```python
from build123d import *

# Parameters (mm, degrees)
SKETCH4_W           = 60
SKETCH4_H           = 40
BOSS_EXTRUDE1_DEPTH = 20
FILLET1_R           = 5
FILLET2_R           = 5
CUT_EXTRUDE1_DEPTH  = 8
CUT_EXTRUDE2_DEPTH  = 8
SKETCH8_R           = 1.5
CUT_EXTRUDE4_DEPTH  = 8
SHELL3_START        = 2
SHELL3_DEPTH        = 18
SKETCH9_W           = 10.049922194
SKETCH9_H           = 4.5
BOSS_EXTRUDE2_DEPTH = 1
SKETCH10_W          = 0.584985694
SKETCH10_H          = 1.811393404
CUT_EXTRUDE5_DEPTH  = 0.1
CUT_EXTRUDE6_DEPTH  = 5.1


# Read off the part's stored shape, not the designer's step: Shell3
with BuildPart() as part:
    # Sketch4 → Boss-Extrude1 (new body)
    with BuildSketch(Plane(origin=(0, 0, 0), x_dir=(1, 0, 0), z_dir=(0, 1, 0))):
        with Locations((-9.826955075, -12.370810554)):
            Rectangle(SKETCH4_W, SKETCH4_H)
    extrude(amount=BOSS_EXTRUDE1_DEPTH)

    # Fillet1
    fillet1_edges = [part.edges().sort_by_distance(p)[0] for p in [
        (20.173044925, 10, 32.370810554),
    ]]
    fillet(fillet1_edges, radius=FILLET1_R)

    # Fillet2
    fillet2_edges = [part.edges().sort_by_distance(p)[0] for p in [
        (20.173044925, 10, -7.629189446),
        (-39.826955075, 10, 32.370810554),
    ]]
    fillet(fillet2_edges, radius=FILLET2_R)

    # Sketch6 → Cut-Extrude1 (cut)
    with BuildSketch(Plane(origin=(0, 20, 0), x_dir=(1, 0, 0), z_dir=(0, 1, 0))):
        Polygon((-32.326955075, 7.629189446), (-39.826955075, 0.129189446), (-39.826955075, 7.629189446), align=None)
    extrude(amount=-CUT_EXTRUDE1_DEPTH, mode=Mode.SUBTRACT)

    # Sketch7 → Cut-Extrude2 (cut)
    with BuildSketch(Plane.XZ):
        Polygon((-32.326955075, -7.629189446), (-39.826955075, -0.129189446), (-39.826955075, -7.629189446), align=None)
    extrude(amount=-CUT_EXTRUDE2_DEPTH, mode=Mode.SUBTRACT)

    # Sketch8 → Cut-Extrude4 (cut)
    with BuildSketch(Plane(origin=(0, 12, 0), x_dir=(1, 0, 0), z_dir=(0, 1, 0))):
        with Locations(Location((-37.501831714, 5.285439446, 0), (0, 0, 270))):
            Circle(SKETCH8_R)
    extrude(amount=-CUT_EXTRUDE4_DEPTH, mode=Mode.SUBTRACT)

    # Shell3 outline → Shell3 (cut)
    with BuildSketch(Plane(origin=(0, 0, 0), x_dir=(1, 0, 0), z_dir=(0, 1, 0)).offset(SHELL3_START)):
        with BuildLine():
            Line((-37.826955075, -0.699237679), (-37.826955075, -27.370810554))
            ThreePointArc((-37.826955075, -27.370810554), (-36.948275418, -29.492130897), (-34.826955075, -30.370810554))
            Line((-34.826955075, -30.370810554), (15.173044925, -30.370810554))
            ThreePointArc((15.173044925, -30.370810554), (17.294365268, -29.492130897), (18.173044925, -27.370810554))
            Line((18.173044925, -27.370810554), (18.173044925, 2.629189446))
            ThreePointArc((18.173044925, 2.629189446), (17.294365269, 4.75050979), (15.173044925, 5.629189446))
            Line((15.173044925, 5.629189446), (-31.49852795, 5.629189446))
            Line((-31.49852795, 5.629189446), (-37.826955075, -0.699237679))
        make_face()
    extrude(amount=SHELL3_DEPTH, mode=Mode.SUBTRACT)

    # Sketch9 → Boss-Extrude2 (add)
    with BuildSketch(Plane.XY.offset(32.370810554)):
        with Locations((2.673044925, 10)):
            Rectangle(SKETCH9_W, SKETCH9_H)
    extrude(amount=BOSS_EXTRUDE2_DEPTH)

    # Sketch10 → Cut-Extrude5 (cut)
    with BuildSketch(Plane.XY.offset(33.370810554)):
        with BuildLine():
            Line((1.902705655, 11.169007018), (1.738142725, 11.418734932))
            ThreePointArc((1.738142725, 11.418734932), (2.673044925, 8.300926449), (3.607947125, 11.418734932))
            Line((3.607947125, 11.418734932), (3.443384196, 11.169007018))
            ThreePointArc((3.443384196, 11.169007018), (2.673044925, 8.6), (1.902705655, 11.169007018))
        make_face()
        with Locations((2.673044925, 11.125)):
            Rectangle(SKETCH10_W, SKETCH10_H)
    extrude(amount=-CUT_EXTRUDE5_DEPTH, mode=Mode.SUBTRACT)

    # Sketch11 → Cut-Extrude6 (cut)
    with BuildSketch(Plane.XY.offset(32.370810554)):
        Polygon((-13.276955075, 10), (-13.276955075, 11.1), (-6.376955075, 11.1), (-6.376955075, 10), (-7.126955075, 9.25), (-9.826955075, 9.25), (-12.526955075, 9.25), align=None)
    extrude(amount=-CUT_EXTRUDE6_DEPTH, mode=Mode.SUBTRACT)


solid = part.part
```
The listing builds one solid part. Answer for the finished solid, in the listing's coordinates (mm). A direction names the side the tool comes from. Give positions to 0.01 mm unless a question says otherwise; leave off trailing zeros. Loops run counter-clockwise (first coordinate to the right, second up) from the corner with the lowest first, then second, coordinate; pieces in that order, holes last. Notation, with made-up numbers: (73, 36.5) - (129, 36.5) arc R32 ccw to (129, 67.5) - close; hole circle Ø5 at (35, -4.5). An arc over 180 degrees is marked (long way). Return JSON: item names as keys, results as strings. Group by question number.
1. Find section B-B (x = 9.5). Write down the section's boundary in (y, z), then the cut area to 3 significant figures.
2. Given pin 1 Ø0.6 at (x, z) = (-11.5, 31.5) entering from -Y; pin 2 Ø1.1 at (y, z) = (9.5, 33) entering from -X; pin 3 Ø1.5 at (x, z) = (-27, 25) entering from +Y, each flat-ended and moving along its own axis, determine where each tip first touches the part or whether it passes through.
3. Which of the six approach directions +Z, -Z, +X, -X, +Y, -Y give full straight-line access (tool end or side, diameter ignored) to faces 5 (the flat face through (-13, 10, -7.629)), 6 (the cylindrical face through (-36.97, 10.87, 29.47)), 7 (the flat face through (-35.8, 12, -5.3)), 8 (the flat face through (-10, 9.25, 31))?
4. Find section A-A (y = 6.75). Write down the section's boundary in (x, z), then the cut area to 3 significant figures.
5. Determine the mould class of faces 1 (the flat face through (-39.827, 10, 14)), 2 (the cylindrical face through (18.747, 10.14, -6.126)), 3 (the cylindrical face through (-36.5, 10, -6.4)), 4 (the cylindrical face through (18.669, 10.14, 30.945)) for opening direction Z: pulls with the +Z half, pulls with the -Z half, needs draft (parallel to the pull), parting line crosses it, or undercut.
6. Find section C-C (z = 11.5). Write down the section's boundary in (x, y).
7. Straight lines are drawn through the part: line 1 (X direction, y = 18, z = 21.5); line 2 (Z direction, x = -25.5, y = 9); line 3 (Y direction, x = -21, z = 21.5). For each, find the intervals that lie inside material, in ascending order. Write a range as [from, to].
Verdict:
{
 "1": {"outline": "(0, -7.63) - (20, -7.63) - (20, -5.63) - (2, -5.63) - (2, 30.37) - (20, 30.37) - (20, 32.37) - (0, 32.37) - close", "area": "152 mm^2"},
 "2": {"pin 1": "stops at y = 0", "pin 2": "stops at x = -2.35", "pin 3": "stops at y = 2"},
 "3": {"face 5": "-Z, +X, -X, +Y, -Y", "face 6": "+Y", "face 7": "-Z, -X, +Y", "face 8": "+Z"},
 "4": {"outline": "(-39.83, -0.13) - (-32.33, -7.63) - (15.17, -7.63) arc R5 ccw to (20.17, -2.63) - (20.17, 27.37) arc R5 ccw to (15.17, 32.37) - (-34.83, 32.37) arc R5 ccw to (-39.83, 27.37) - close; hole (-37.83, 0.7) - (-31.5, -5.63) - (15.17, -5.63) arc R3 ccw to (18.17, -2.63) - (18.17, 27.37) arc R3 ccw to (15.17, 30.37) - (-34.83, 30.37) arc R3 ccw to (-37.83, 27.37) - close", "area": "366 mm^2"},
 "5": {"face 1": "needs draft", "face 2": "pulls with the -Z half", "face 3": "undercut", "face 4": "pulls with the +Z half"},
 "6": {"outline": "(-39.83, 0) - (20.17, 0) - (20.17, 20) - (18.17, 20) - (18.17, 2) - (-37.83, 2) - (-37.83, 20) - (-39.83, 20) - close"},
 "7": {"line 1": "x = [-39.83, -37.83], [18.17, 20.17]", "line 2": "z = [-7.63, -5.63], [30.37, 32.37]", "line 3": "y = [0, 2]"}
}
